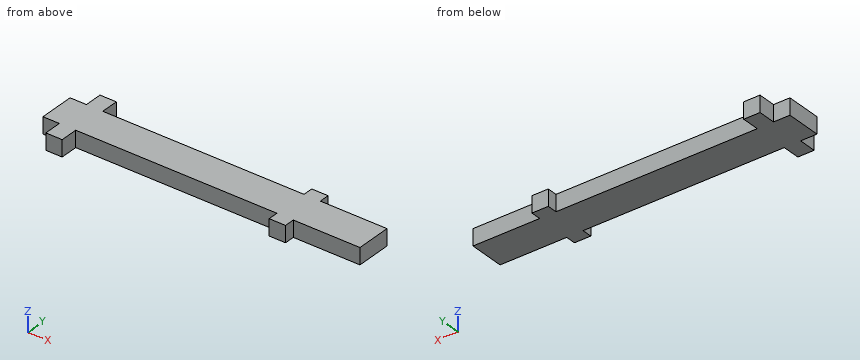
Autodesk Inventor part; units mm, degrees
ref_plane "YZ Plane" through (0, 0, 0) normal (1, 0, 0) x (0, 1, 0)
ref_plane "XZ Plane" through (0, 0, 0) normal (0, 1, 0) x (-1, 0, 0)
ref_plane "XY Plane" through (0, 0, 0) normal (0, 0, 1) x (1, 0, 0)
sketch "Sketch1" plane through (0, 0, 0) normal (0, 0, 1) x (1, 0, 0)
  line L0 (-92.7646, -8.503) -> (-89.7646, -8.503)
  line L1 (-89.7646, -8.503) -> (-89.7646, -11.753)
  line L2 (-89.7646, -11.753) -> (-92.7646, -11.753)
  line L3 (-92.7646, -11.753) -> (-92.7646, -8.503)
  line L4 (-92.7646, -21.6527) -> (-89.7646, -21.6527)
  line L5 (-89.7646, -21.6527) -> (-89.7646, -21.7527)
  line L6 (-89.7646, -21.7527) -> (-92.7646, -21.7527)
  line L7 (-92.7646, -21.7527) -> (-92.7646, -21.6527)
  line L8 (-70.621, 23.5389) -> (-20.621, 23.5389)
  line L9 (-20.621, 23.5389) -> (-20.621, 16.5389)
  line L10 (-20.621, 16.5389) -> (-70.621, 16.5389)
  line L11 (-70.621, 16.5389) -> (-70.621, 23.5389)
  line L12 (-73.871, 27.0389) -> (-70.621, 27.0389)
  line L13 (-70.621, 27.0389) -> (-70.621, 13.0389)
  line L14 (-70.621, 13.0389) -> (-73.871, 13.0389)
  line L15 (-73.871, 13.0389) -> (-73.871, 27.0389)
  line L16 (-73.871, 20.0389) -> (-70.621, 20.0389) construction
  line L17 (-20.621, 20.0389) -> (-70.621, 20.0389) construction
  line L18 (-45.621, 23.5389) -> (-45.621, 16.5389) construction
  line L19 (-77.121, 23.5389) -> (-73.871, 23.5389)
  line L20 (-73.871, 23.5389) -> (-73.871, 16.5389)
  line L21 (-73.871, 16.5389) -> (-77.121, 16.5389)
  line L22 (-77.121, 16.5389) -> (-77.121, 23.5389)
  line L23 (-77.121, 20.0389) -> (-73.871, 20.0389) construction
  line L24 (-20.621, 23.5389) -> (-17.371, 23.5389)
  line L25 (-17.371, 23.5389) -> (-17.371, 16.5389)
  line L26 (-17.371, 16.5389) -> (-20.621, 16.5389)
  line L27 (-20.621, 16.5389) -> (-20.621, 23.5389)
  line L28 (-14.121, 23.5389) -> (-17.371, 23.5389)
  line L29 (-17.371, 23.5389) -> (-17.371, 16.5389)
  line L30 (-17.371, 16.5389) -> (-14.121, 16.5389)
  line L31 (-14.121, 16.5389) -> (-14.121, 23.5389)
  line L32 (-14.121, 20.0389) -> (-17.371, 20.0389) construction
  line L33 (-30.621, 25.5389) -> (-27.371, 25.5389)
  line L34 (-27.371, 25.5389) -> (-27.371, 14.5389)
  line L35 (-27.371, 14.5389) -> (-30.621, 14.5389)
  line L36 (-30.621, 14.5389) -> (-30.621, 25.5389)
  line L37 (-30.621, 20.0389) -> (-27.371, 20.0389) construction
  point P0 (0, 0)
  point P1 (-17.371, 20.0389)
  dimension "d3" = 3
  dimension "mat" = 3.25
  dimension "d5" = 3
  dimension "kerf" = 0.1
  dimension "d44" = 3.25
  dimension "d45" = 14
  dimension "d46" = 3.25
  dimension "d47" = 7
  dimension "d48" = 50
  dimension "d49" = 3.25
  dimension "d50" = 7
  dimension "d53" = 3.25
  dimension "d54" = 11
  dimension "d55" = 40
extrude "Extrusion6" add sketch "Sketch1" along normal blind 3.25 contours L8 L36 L10 L11 | L11 L13 L14 L15 L12 | L8 L34 L10 L36 | L8 L9 L10 L34 | L24 L25 L26 L9 | L15 L21 L22 L19 | L28 L31 L30 L25
extrude "Extrusion7" add sketch "Sketch1" along normal blind 3.25 contours L36 L33 L34 L8 | L8 L34 L10 L36 | L10 L34 L35 L36
equation "\"d44\" = mat"
equation "\"d46\" = mat"
equation "\"d49\" = mat"
equation "\"d53\" = mat"
equation "\"d51\" = mat"
equation "\"d56\" = mat"
properties part number "body-back"
For this review, take the finished solid that the model builds, in its own axes (mm). Coordinates: 2 decimals unless noted, no trailing zeros. Loops run counter-clockwise (first coordinate to the right, second up) from the corner with the lowest first, then second, coordinate; pieces in that order, holes last. Notation, with made-up numbers: (20, 34.5) - (41, 34.5) arc R28 ccw to (41, 60.5) - close; hole circle Ø10 at (34.5, -27). An arc over 180 degrees is marked (long way). Use one line per item in the form item = value. Start each with the question number.
1) For pin 1 (1.6 mm diameter, centred on y = 24.5, z = 1.5, fed in from -X); pin 2 (8 mm diameter, centred on x = -52.5, y = 25, fed in from +Z); pin 3 (1 mm diameter, centred on x = -21, z = 1.5, fed in from -Y); pin 4 (1 mm diameter, centred on x = -18, z = 1.5, fed in from +Y), all flat-tipped, find the tip position at first contact; note any pin that passes through.
2) Take a section at C-C (x = -68). State the section outline as (y, z) points, plus the area to 4 significant figures.
3) Take a section at A-A (y = 24.75). State the section outline as (x, z) points, plus the area to 3 significant figures.
4) To check wall thickness, follow probe 1 along X at (y, z) = (15.75, 2.55); probe 2 along Y at (x, z) = (-22, 0.35); probe 3 along X at (y, z) = (13.75, 1.3). State the ranges of each line that lie inside material, in increasing order. Write a range as from..to.
5) Take a section at B-B (z = 2). State the section outline as (x, y) points, plus the area to 3 significant figures.
From the geometry:
q1.pin_1 = -73.87
q1.pin_2 = 3.25
q1.pin_3 = 16.54
q1.pin_4 = 23.54
q2.outline = (16.54, 0) - (23.54, 0) - (23.54, 3.25) - (16.54, 3.25) - close
q2.area = 22.75 mm2
q3.outline = (-73.87, 0) - (-70.62, 0) - (-70.62, 3.25) - (-73.87, 3.25) - close; (-30.62, 0) - (-27.37, 0) - (-27.37, 3.25) - (-30.62, 3.25) - close
q3.area = 21.1 mm2
q4.probe_1 = -73.87..-70.62, -30.62..-27.37
q4.probe_2 = 16.54..23.54
q4.probe_3 = -73.87..-70.62
q5.outline = (-77.12, 16.54) - (-73.87, 16.54) - (-73.87, 13.04) - (-70.62, 13.04) - (-70.62, 16.54) - (-30.62, 16.54) - (-30.62, 14.54) - (-27.37, 14.54) - (-27.37, 16.54) - (-14.12, 16.54) - (-14.12, 23.54) - (-27.37, 23.54) - (-27.37, 25.54) - (-30.62, 25.54) - (-30.62, 23.54) - (-70.62, 23.54) - (-70.62, 27.04) - (-73.87, 27.04) - (-73.87, 23.54) - (-77.12, 23.54) - close
q5.area = 477 mm2
